Autodesk Inventor part; units mm, degrees
ref_plane "Start plane" through (0, 0, -17.5) normal (0, 0, 1) x (1, 0, 0)
ref_plane "End plane" through (0, 0, 405.5) normal (0, 0, 1) x (1, 0, 0)
ref_plane "Work Plane11" through (-8.5964, 0, 403.2431) normal (-0.4912, 0, 0.871) x (0.871, 0, 0.4912)
ref_plane "Start plane" through (0, 0, -17.5) normal (0, 0, 1) x (1, 0, 0)
ref_plane "End plane" through (0, 0, 405.5) normal (0, 0, 1) x (1, 0, 0)
sketch "Sketch" plane through (0, 0, 0) normal (0, 0, 1) x (1, 0, 0)
  line L0 (-17.5, -14.3) -> (-17.5, 14.3)
  line L1 (-14.3, 17.5) -> (14.3, 17.5)
  line L2 (17.5, 14.3) -> (17.5, -14.3)
  line L3 (14.3, -17.5) -> (-14.3, -17.5)
  arc A0 (-17.5, -14.3) -> (-14.3, -17.5) centre (-14.3, -14.3) ccw
  arc A1 (-14.3, 17.5) -> (-17.5, 14.3) centre (-14.3, 14.3) ccw
  arc A2 (17.5, 14.3) -> (14.3, 17.5) centre (14.3, 14.3) ccw
  arc A3 (14.3, -17.5) -> (17.5, -14.3) centre (14.3, -14.3) ccw
  arc A4 (-14.3, 15.9) -> (-15.9, 14.3) centre (-14.3, 14.3) ccw
  line L4 (-14.3, 15.9) -> (14.3, 15.9)
  arc A5 (15.9, 14.3) -> (14.3, 15.9) centre (14.3, 14.3) ccw
  line L5 (15.9, 14.3) -> (15.9, -14.3)
  arc A6 (14.3, -15.9) -> (15.9, -14.3) centre (14.3, -14.3) ccw
  line L6 (14.3, -15.9) -> (-14.3, -15.9)
  arc A7 (-15.9, -14.3) -> (-14.3, -15.9) centre (-14.3, -14.3) ccw
  line L7 (-15.9, -14.3) -> (-15.9, 14.3)
  line L8 (0, 25.4278) -> (0, -25.4278) construction
  line L9 (-25.4278, 0) -> (25.4278, 0) construction
  dimension "d7" = 3.2
  dimension "d10" = 35
  dimension "d11" = 35
  dimension "d12" = 1.6
  dimension "d15" = 17.5
  dimension "d16" = 17.5
extrude "Body" add sketch "Sketch" along normal up to surface (423 mm away) from surface at -17.5
sketch "Sketch3" plane through (0, 0, 0) normal (0, 0, 1) x (1, 0, 0)
  line L0 (0, 0) -> (10, 0)
ref_plane "Work Plane3" through (0, 0, 0) normal (0, -1, 0) x (1, 0, 0)
sketch "Sketch4" plane through (0, 0, 0) normal (0, -1, 0) x (1, 0, 0)
  line L0 (-2, -17.5) -> (12, -17.5)
  line L1 (-2, 405.5) -> (12, 405.5)
  dimension "d18" = 423
ref_plane "Work Plane11" through (-8.5964, 0, 403.2431) normal (-0.4912, 0, 0.871) x (0.871, 0, 0.4912)
split "Split5" plane through (-8.5964, 0, 403.2431) removes the side toward (-0.4912, 0, 0.871)
ref_plane "Work Plane12" through (-696.5964, 0, 372.7569) normal (-0.4912, 0, -0.871) x (-0.871, 0, 0.4912)
split "Split6" plane through (-696.5964, 0, 372.7569) removes the side toward (-0.4912, 0, -0.871)
ref_plane "Work Plane13" through (17.5, 0, 405.5) normal (-0.7071, 0, 0.7071) x (0.7071, 0, 0.7071)
split "Split7" plane through (17.5, 0, 405.5) removes the side toward (-0.7071, 0, 0.7071)
ref_plane "Work Plane14" through (17.5, 0, -17.5) normal (-0.7071, 0, -0.7071) x (-0.7071, 0, 0.7071)
split "Split8" plane through (17.5, 0, -17.5) removes the side toward (-0.7071, 0, -0.7071)
equation "\"d7\" = G_IR"
equation "\"d10\" = G_H"
equation "\"d11\" = G_W"
equation "\"d12\" = G_T"
equation "\"d15\" = 0.5 * d10"
equation "\"d16\" = 0.5 * d11"
equation "\"d3\" = G_L"
equation "\"G_W\" = 35"
equation "\"G_H\" = 35"
equation "\"G_T\" = 1.6"
equation "\"G_IR\" = 3.2"
equation "\"G_L\" = d18"
equation "\"G_OFFSET_START\" = 17.5"
equation "\"G_OFFSET_END\" = 17.5"
equation "\"d13\" = -G_OFFSET_START"
equation "\"d14\" = G_OFFSET_END + B_L"
equation "\"B_L\" = 388"
properties part number "AS 1163 - C350L0 35x35x1.6 SHS - 423" material "Steel, Mild"
Could you check a few things on this model? Use its own coordinates, in mm. A direction names the side the tool comes from. Coordinates: 2 decimals unless noted, no trailing zeros. Order: outer loops, then holes, each group sorted by start corner. A loop starts at its lowest first (then second) coordinate and runs counter-clockwise, first axis right, second up. Notation, with made-up numbers: M 26.25,-20.75 L 39.25,-20.75 A19 cw 39.25,-13.75 Z; hole C 67.5,-15 d1. An arc over 180 degrees is marked long. Use one line per item in the form item = value. Start each with the question number.
1. Please list where these lines run through material, in increasing order: line 1 (Y direction, x = 2, z = 342); line 2 (Y direction, x = -15.5, z = 293.5).
2. We'd pull the mould along X, two halves only. Please class faces 1 (the flat face through (0, 17, 0)), 2 (the flat face through (0, -15.9, 191)), 3 (the flat face through (0, 17.5, 191)): +X half, -X half, draft (parallel to the pull), parting line (faces both ways), or undercut.
3. Suppose I cut it at B-B on x = 0.5. Write out the boundary of the cut face in (y, z), then the cut area to 3 significant figures.
4. On a 3-axis mill with a long thin cutter (end or side, diameter ignored), from which of +Z, -Z, +X, -X, +Y, -Y can I reach the whole of each face in a straight line? I mean faces 4 (the flat face through (15.9, 0, 191)), 5 (the flat face through (17.5, 0, 191)). Say none if no direction works.
5. Suppose I cut it at A-A on y = -8. Write out the boundary of the cut face in (x, z).
6. Suppose I cut it at C-C on z = 284. Write out the boundary of the cut face in (x, y).
7. For pin 1 (12 mm diameter, centred on x = 10, y = -2, fed in from +Z); pin 2 (10 mm diameter, centred on x = -4.5, y = -14, fed in from -Z), each with a flat end and sliding along its axis, tell me the tip position at first contact or that it passes through.
Geometry says:
q1.line_1 = -17.5 to -15.9, 15.9 to 17.5
q1.line_2 = -17.27 to -15.36, 15.36 to 17.27
q2.face_1 = -X half
q2.face_2 = undercut
q2.face_3 = draft
q3.outline = M -17.5,-0.5 L -15.9,-0.5 L -15.9,388.5 L -17.5,388.5 Z; M 15.9,-0.5 L 17.5,-0.5 L 17.5,388.5 L 15.9,388.5 Z
q3.area = 1,240 mm^2
q4.face_4 = +Z, -Z
q4.face_5 = +Z, -Z, +X, +Y, -Y
q5.outline = M -17.5,17.5 L -15.9,15.9 L -15.9,372.1 L -17.5,370.5 Z; M 15.9,-15.9 L 17.5,-17.5 L 17.5,405.5 L 15.9,403.9 Z
q6.outline = M -17.5,-14.3 A3.2 ccw -14.3,-17.5 L 14.3,-17.5 A3.2 ccw 17.5,-14.3 L 17.5,14.3 A3.2 ccw 14.3,17.5 L -14.3,17.5 A3.2 ccw -17.5,14.3 Z; hole M -15.9,-14.3 A1.6 ccw -14.3,-15.9 L 14.3,-15.9 A1.6 ccw 15.9,-14.3 L 15.9,14.3 A1.6 ccw 14.3,15.9 L -14.3,15.9 A1.6 ccw -15.9,14.3 Z
q7.pin_1 = 404
q7.pin_2 = -0.12
